```python
from build123d import *

# Parameters (mm, degrees)
CROQUIS1_R                   = 3.97256
SALIENTE_EXTRUIR2_DEPTH      = 5.08
CROQUIS2_R                   = 1.524
SALIENTE_EXTRUIR4_DEPTH      = 177.8
SALIENTE_EXTRUIR4_DEPTH_BACK = 2.54
CROQUIS3_R                   = 4.149655304
CORTAR_EXTRUIR1_DEPTH        = 20.32
CORTAR_EXTRUIR1_DEPTH_BACK   = 21.336


with BuildPart() as part:
    # Croquis1 → Saliente-Extruir2 (new body)
    with BuildSketch(Plane(origin=(0, 0, 0), x_dir=(1, 0, 0), z_dir=(0, 1, 0))):
        Polygon((6.921319842, 0), (3.460659921, 5.994038811), (-3.460659921, 5.994038811), (-6.921319842, 0), (-3.460659921, -5.994038811), (3.460659921, -5.994038811), align=None)
        Circle(CROQUIS1_R, mode=Mode.SUBTRACT)
    extrude(amount=SALIENTE_EXTRUIR2_DEPTH)

    # Croquis2 → Saliente-Extruir4 (add, two sides)
    with BuildSketch(Plane.XY) as saliente_extruir4_sk:
        with Locations((0, 2.54)):
            Circle(CROQUIS2_R)
    extrude(amount=SALIENTE_EXTRUIR4_DEPTH)
    extrude(saliente_extruir4_sk.sketch, amount=-SALIENTE_EXTRUIR4_DEPTH_BACK)

    # Croquis3 → Cortar-Extruir1 (cut, two sides)
    with BuildSketch(Plane(origin=(0, 0, 0), x_dir=(1, 0, 0), z_dir=(0, 1, 0))) as cortar_extruir1_sk:
        Circle(CROQUIS3_R)
    extrude(amount=CORTAR_EXTRUIR1_DEPTH, mode=Mode.SUBTRACT)
    extrude(cortar_extruir1_sk.sketch, amount=-CORTAR_EXTRUIR1_DEPTH_BACK, mode=Mode.SUBTRACT)


solid = part.part
```
Read the model definition and answer for the solid it produces. Units are mm, in the model's axes. A direction names the side the tool comes from. Give positions to 0.01 mm unless a question says otherwise; leave off trailing zeros. Write each loop counter-clockwise with the first axis right and the second up, starting at its lowest first coordinate (ties: lowest second). Pieces come first, ordered by that corner, then holes. Notation, with made-up numbers: (-25.75, 4) -> (0.25, 4) arc R16 cw to (0.25, 26) -> close; hole circle Ø2 at (3.25, 44.25). An arc over 180 degrees is marked (long way). Answer in a Markdown table with one row per item.
1) Section C-C on z = 158 is taken. Give the vertices of the cut face in (x, y), plus the area to 3 significant figures.
Results list:
| item | result |
|---|---|
| outline | circle Ø3.05 at (0, 2.54) |
| area | 7.30 mm^2 |
2) Each of these flat-tipped pins is pushed along its axis until it touches: pin 1 Ø3 at (y, z) = (3, 76.5) entering from -X; pin 2 Ø3 at (x, z) = (-1.5, 49) entering from -Y; pin 3 Ø1 at (x, z) = (1.5, 80.5) entering from +Y. Where does it stop, or does it pass through?
Results list:
| item | result |
|---|---|
| pin 1 | x = -1.52 |
| pin 2 | y = 1.02 |
| pin 3 | y = 3.69 |
3) A tool of negligible diameter and unlimited length cuts with its end or side. For faces 1 (the flat face through (-2, 3, 5.994)), 2 (the flat face through (0, 3, -5.994)), from which of +Z, -Z, +X, -X, +Y, -Y can it reach the whole face along a straight path? Write none if from no direction.
Results list:
| item | result |
|---|---|
| face 1 | +Z |
| face 2 | -Z, +X, -X, +Y, -Y |
4) Section A-A on x = 0 is taken. Give the vertices of the cut face in (y, z), plus the area to 3 significant figures.
Results list:
| item | result |
|---|---|
| outline | (0, -5.99) -> (5.08, -5.99) -> (5.08, -4.15) -> (0, -4.15) -> close; (0, 4.15) -> (5.08, 4.15) -> (5.08, 5.99) -> (4.06, 5.99) -> (4.06, 177.8) -> (1.02, 177.8) -> (1.02, 5.99) -> (0, 5.99) -> close |
| area | 542 mm^2 |
5) Determine the mould class of faces 3 (the cylindrical face through (-0.33, 1.052, 90.694)), 4 (the cylindrical face through (-3.29, 2.5, 2.53)), 5 (the flat face through (1.4, 5.08, -4.1)), 6 (the flat face through (-5.167, 2.504, -3.039)) for opening direction X: released by +X, released by -X, zero draft, split by the parting line, or undercut.
Results list:
| item | result |
|---|---|
| face 3 | split by the parting line |
| face 4 | undercut |
| face 5 | zero draft |
| face 6 | released by -X |
6) Straight lines are drawn through the part: line 1 (X direction, y = 1.8, z = 0); line 2 (Z direction, x = 0, y = 2.9); line 3 (Z direction, x = -2.25, y = 3.75). For each, find the intervals that lie inside material, in ascending order. Write a range as [from, to].
Results list:
| item | result |
|---|---|
| line 1 | [-6.92, -4.15], [4.15, 6.92] |
| line 2 | [-5.99, -4.15], [4.15, 177.8] |
| line 3 | [-5.99, -3.49], [3.49, 5.99] |
7) Section B-B on y = 2.54 is taken. Give the vertices of the cut face in (x, z).
Results list:
| item | result |
|---|---|
| outline | (-6.92, 0) -> (-3.46, -5.99) -> (3.46, -5.99) -> (6.92, 0) -> (3.46, 5.99) -> (1.52, 5.99) -> (1.52, 177.8) -> (-1.52, 177.8) -> (-1.52, 5.99) -> (-3.46, 5.99) -> close; hole circle Ø8.3 at (0, 0) |
